Geometry: final body of the model. Coordinates: model frame, mm. A direction names the side the tool comes from. Give positions to 0.01 mm unless a question says otherwise; leave off trailing zeros. Loops run counter-clockwise (first coordinate to the right, second up) from the corner with the lowest first, then second, coordinate; pieces in that order, holes last. Notation, with made-up numbers: (-35, 89) - (8, 89) arc R17 ccw to (8, 111) - close; hole circle Ø9 at (40, 72.25). An arc over 180 degrees is marked (long way). Answer in a Markdown table with one row per item.
from build123d import *

# Parameters (mm, degrees)
SKETCH1_W                  = 56.4
SKETCH1_H                  = 56.4
BOSS_EXTRUDE1_DEPTH        = 86
SKETCH2_W                  = 9.63
SKETCH2_H                  = 9.63
CUT_EXTRUDE1_DEPTH         = 81.2
FILLET1_R                  = 5
FILLET2_R                  = 2.4
FILLET3_R                  = 4.6
F_5_1_5_1_DIAMETER_HOLE1_D = 5.1
CIRPATTERN1_COUNT          = 4
SKETCH7_R                  = 19.05
BOSS_EXTRUDE2_DEPTH        = 1.6
SKETCH8_R                  = 3.175
BOSS_EXTRUDE3_DEPTH        = 19
CUT_EXTRUDE2_START         = -15
CUT_EXTRUDE2_DEPTH         = 15
SKETCH11_W                 = 32.34
SKETCH11_H                 = 20
BOSS_EXTRUDE4_DEPTH        = 0.2


with BuildPart() as part:
    # Sketch1 → Boss-Extrude1 (new body)
    with BuildSketch(Plane.XY):
        Rectangle(SKETCH1_W, SKETCH1_H)
    extrude(amount=-BOSS_EXTRUDE1_DEPTH)

    # Sketch2 → Cut-Extrude1 (cut)
    with BuildSketch(Plane(origin=(0, 0, -86), x_dir=(-1, 0, 0), z_dir=(0, 0, -1))):
        with Locations((23.385, 23.385)):
            Rectangle(SKETCH2_W, SKETCH2_H)
        with Locations((-23.385, 23.385)):
            Rectangle(SKETCH2_W, SKETCH2_H)
        with Locations((23.385, -23.385)):
            Rectangle(SKETCH2_W, SKETCH2_H)
        with Locations((-23.385, -23.385)):
            Rectangle(SKETCH2_W, SKETCH2_H)
    extrude(amount=-CUT_EXTRUDE1_DEPTH, mode=Mode.SUBTRACT)

    # Fillet1
    fillet1_edges = [part.edges().sort_by_distance(p)[0] for p in [
        (18.57, -18.57, -45.4),
        (-18.57, -18.57, -45.4),
        (-18.57, 18.57, -45.4),
        (18.57, 18.57, -45.4),
    ]]
    fillet(fillet1_edges, radius=FILLET1_R)

    # Fillet2
    fillet2_edges = [part.edges().sort_by_distance(p)[0] for p in [
        (18.57, -28.2, -45.4),
        (28.2, -18.57, -45.4),
        (-28.2, -18.57, -45.4),
        (-18.57, -28.2, -45.4),
        (-18.57, 28.2, -45.4),
        (-28.2, 18.57, -45.4),
        (28.2, 18.57, -45.4),
        (18.57, 28.2, -45.4),
    ]]
    fillet(fillet2_edges, radius=FILLET2_R)

    # Fillet3
    fillet3_edges = [part.edges().sort_by_distance(p)[0] for p in [
        (28.2, 28.2, -2.4),
        (-28.2, 28.2, -2.4),
        (-28.2, -28.2, -2.4),
        (28.2, -28.2, -2.4),
    ]]
    fillet(fillet3_edges, radius=FILLET3_R)

    # Ø5.1 (5.1) Diameter Hole1 (through all)
    with Locations(Plane.XY):
        with Locations((-23.57, 23.57)):
            f_5_1_5_1_diameter_hole1 = Hole(F_5_1_5_1_DIAMETER_HOLE1_D / 2)

    # CirPattern1: Ø5.1 (5.1) Diameter Hole1 ×4 about axis
    cirpattern1_axis = Axis((0, 0, 0), (0, 0, 1))
    for i in range(1, CIRPATTERN1_COUNT):
        add(f_5_1_5_1_diameter_hole1.rotate(cirpattern1_axis, i * 360 / CIRPATTERN1_COUNT), mode=Mode.SUBTRACT)

    # Sketch7 → Boss-Extrude2 (add)
    with BuildSketch(Plane.XY):
        Circle(SKETCH7_R)
    extrude(amount=BOSS_EXTRUDE2_DEPTH)

    # Sketch8 → Boss-Extrude3 (add)
    with BuildSketch(Plane.XY.offset(1.6)):
        Circle(SKETCH8_R)
    extrude(amount=BOSS_EXTRUDE3_DEPTH)

    # Sketch9 → Cut-Extrude2 (cut)
    with BuildSketch(Plane.XY.offset(20.6).offset(CUT_EXTRUDE2_START)):
        with BuildLine():
            Line((-1.71, 2.675168219), (1.71, 2.675168219))
            ThreePointArc((1.71, 2.675168219), (0, 3.175), (-1.71, 2.675168219))
        make_face()
    extrude(amount=CUT_EXTRUDE2_DEPTH, mode=Mode.SUBTRACT)

    # Sketch11 → Boss-Extrude4 (add)
    with BuildSketch(Plane.XZ.offset(28.2)):
        with Locations((0, -76)):
            Rectangle(SKETCH11_W, SKETCH11_H)
        with Locations((0, -14.8)):
            Rectangle(SKETCH11_W, SKETCH11_H)
    extrude(amount=BOSS_EXTRUDE4_DEPTH)


solid = part.part
Q1. Reachability of faces 1 (the flat face through (0, -28.2, -2)), 2 (the flat face through (-19.2, 0.4, 0)), 3 (the flat face through (-25, 18.57, -46)), 4 (the flat face through (23.6, -20.8, -4.8)) from +Z, -Z, +X, -X, +Y, -Y: full face, straight path, thin tool, end or side. Return the list, or none.
Check values:
| item | result |
|---|---|
| face 1 | +Z, +X, -X, -Y |
| face 2 | +Z |
| face 3 | -Z, -X, +Y |
| face 4 | -Z, +X, -Y |
Q2. Cut plane D-D (z = -10.5). Output: boundary loops of the cut face in (x, y), and give its area (3 significant figures).
Check values:
| item | result |
|---|---|
| outline | (-28.2, -16.17) arc R2.4 ccw to (-25.8, -18.57) - (-23.57, -18.57) arc R5 cw to (-18.57, -23.57) - (-18.57, -25.8) arc R2.4 ccw to (-16.17, -28.2) - (-16.17, -28.4) - (16.17, -28.4) - (16.17, -28.2) arc R2.4 ccw to (18.57, -25.8) - (18.57, -23.57) arc R5 cw to (23.57, -18.57) - (25.8, -18.57) arc R2.4 ccw to (28.2, -16.17) - (28.2, 16.17) arc R2.4 ccw to (25.8, 18.57) - (23.57, 18.57) arc R5 cw to (18.57, 23.57) - (18.57, 25.8) arc R2.4 ccw to (16.17, 28.2) - (-16.17, 28.2) arc R2.4 ccw to (-18.57, 25.8) - (-18.57, 23.57) arc R5 cw to (-23.57, 18.57) - (-25.8, 18.57) arc R2.4 ccw to (-28.2, 16.17) - close |
| area | 2,830 mm² |
Q3. Cut plane C-C (z = -64). Output: boundary loops of the cut face in (x, y), and give its area (3 significant figures).
Check values:
| item | result |
|---|---|
| outline | (-28.2, -16.17) arc R2.4 ccw to (-25.8, -18.57) - (-23.57, -18.57) arc R5 cw to (-18.57, -23.57) - (-18.57, -25.8) arc R2.4 ccw to (-16.17, -28.2) - (16.17, -28.2) arc R2.4 ccw to (18.57, -25.8) - (18.57, -23.57) arc R5 cw to (23.57, -18.57) - (25.8, -18.57) arc R2.4 ccw to (28.2, -16.17) - (28.2, 16.17) arc R2.4 ccw to (25.8, 18.57) - (23.57, 18.57) arc R5 cw to (18.57, 23.57) - (18.57, 25.8) arc R2.4 ccw to (16.17, 28.2) - (-16.17, 28.2) arc R2.4 ccw to (-18.57, 25.8) - (-18.57, 23.57) arc R5 cw to (-23.57, 18.57) - (-25.8, 18.57) arc R2.4 ccw to (-28.2, 16.17) - close |
| area | 2,820 mm² |
Q4. First-contact query: pin 1 (2.5 mm diameter, centred on y = 24.5, z = -59, fed in from +X); pin 2 (5 mm diameter, centred on y = 5, z = 4, fed in from -X); pin 3 (1.8 mm diameter, centred on y = -25, z = -46, fed in from -X). Flat tips, straight axial feed; report the tip coordinate or a pass-through.
Check values:
| item | result |
|---|---|
| pin 1 | x = 18.58 |
| pin 2 | x = -18.56 |
| pin 3 | x = -18.57 |
Q5. Cut plane B-B (x = 0). Output: boundary loops of the cut face in (y, z) (3 decimals).
Check values:
| item | result |
|---|---|
| outline | (-28.4, -86) - (28.2, -86) - (28.2, 0) - (19.05, 0) - (19.05, 1.6) - (3.175, 1.6) - (3.175, 5.6) - (2.675, 5.6) - (2.675, 20.6) - (-3.175, 20.6) - (-3.175, 1.6) - (-19.05, 1.6) - (-19.05, 0) - (-28.2, 0) - (-28.2, -4.8) - (-28.4, -4.8) - (-28.4, -24.8) - (-28.2, -24.8) - (-28.2, -66) - (-28.4, -66) - close |
Q6. Material intervals for line 1 along Y through (x, z) = (-23.57, -2); line 2 along X through (y, z) = (23, -1), sorted ascending.
Check values:
| item | result |
|---|---|
| line 1 | -28.2 to -26.12, -21.02 to 21.02, 26.12 to 28.2 |
| line 2 | -28.2 to -26.06, -21.08 to 21.08, 26.06 to 28.2 |
Q7. Draft query along X for faces 5 (the cylindrical face through (-0.69, -3.1, 10.97)), 6 (the flat face through (0, -28.4, -76)), 7 (the cylindrical face through (-20.07, -20, -44.83)), 8 (the cylindrical face through (-23.02, 21.08, -2.43)). Return one class per face: pulls with the +X half, pulls with the -X half, needs draft (parallel to the pull), parting line crosses it, or undercut.
Check values:
| item | result |
|---|---|
| face 5 | parting line crosses it |
| face 6 | needs draft |
| face 7 | pulls with the -X half |
| face 8 | undercut |
Q8. Cut plane A-A (y = 0). Output: boundary loops of the cut face in (x, z) (3 decimals).
Check values:
| item | result |
|---|---|
| outline | (-28.2, -86) - (28.2, -86) - (28.2, 0) - (19.05, 0) - (19.05, 1.6) - (3.175, 1.6) - (3.175, 20.6) - (-3.175, 20.6) - (-3.175, 1.6) - (-19.05, 1.6) - (-19.05, 0) - (-28.2, 0) - close |
